from build123d import *

# Parameters (mm, degrees)
PAD015_DEPTH    = 1
PAD016_DEPTH    = 3
SKETCH029_R     = 1.6
POCKET012_DEPTH = 5


with BuildPart() as part:
    # Sketch027 → Pad015 (new body)
    with BuildSketch(Plane.XY):
        with BuildLine():
            Line((-54.625, 46.125), (-54.625, -46.125))
            ThreePointArc((-54.625, -46.125), (-54.332107, -46.832107), (-53.625, -47.125))
            Line((-53.625, -47.125), (53.625, -47.125))
            ThreePointArc((53.625, -47.125), (54.332107, -46.832107), (54.625, -46.125))
            Line((54.625, -46.125), (54.625, 46.125))
            ThreePointArc((54.625, 46.125), (54.332107, 46.832107), (53.625, 47.125))
            Line((53.625, 47.125), (-53.625, 47.125))
            ThreePointArc((-53.625, 47.125), (-54.332107, 46.832107), (-54.625, 46.125))
        make_face()
    extrude(amount=PAD015_DEPTH)

    # Sketch028 → Pad016 (join)
    with BuildSketch(Plane.XY):
        with BuildLine():
            Line((-54.625, 46.125), (-54.625, -46.125))
            ThreePointArc((-54.625, -46.125), (-54.332107, -46.832107), (-53.625, -47.125))
            Line((-53.625, -47.125), (53.625, -47.125))
            ThreePointArc((53.625, -47.125), (54.332107, -46.832107), (54.625, -46.125))
            Line((54.625, -46.125), (54.625, 46.125))
            ThreePointArc((54.625, 46.125), (54.332107, 46.832107), (53.625, 47.125))
            Line((53.625, 47.125), (-53.625, 47.125))
            ThreePointArc((-53.625, 47.125), (-54.332107, 46.832107), (-54.625, 46.125))
        make_face()
        with BuildLine():
            Line((-53.625, 45.125), (-53.625, -45.125))
            ThreePointArc((-53.625, -45.125), (-53.332107, -45.832107), (-52.625, -46.125))
            Line((-52.625, -46.125), (52.625, -46.125))
            ThreePointArc((52.625, -46.125), (53.332107, -45.832107), (53.625, -45.125))
            Line((53.625, -45.125), (53.625, 45.125))
            ThreePointArc((53.625, 45.125), (53.332107, 45.832107), (52.625, 46.125))
            Line((52.625, 46.125), (-52.625, 46.125))
            ThreePointArc((-52.625, 46.125), (-53.332107, 45.832107), (-53.625, 45.125))
        make_face(mode=Mode.SUBTRACT)
    extrude(amount=-PAD016_DEPTH)

    # Sketch029 → Pocket012 (cut)
    with BuildSketch(Plane.XY):
        with Locations((-48.5, 40)):
            Circle(SKETCH029_R)
        with Locations((-30, 40)):
            Circle(SKETCH029_R)
        with Locations((30, 40)):
            Circle(SKETCH029_R)
        with Locations((-30, -42)):
            Circle(SKETCH029_R)
        with Locations((-48.5, -42)):
            Circle(SKETCH029_R)
        with Locations((30, -42)):
            Circle(SKETCH029_R)
        with Locations((48.5, -42)):
            Circle(SKETCH029_R)
    extrude(amount=POCKET012_DEPTH, mode=Mode.SUBTRACT)


with BuildPart() as part_1:
    # Body007 placement: moved
    add(part.part.moved(Location((0, 0, 36.1))))


solid = part_1.part
Can you work these out from the model? Positions are in its coordinate system, mm. A direction names the side the tool comes from. Give positions to 0.01 mm unless a question says otherwise; leave off trailing zeros. Write each loop counter-clockwise with the first axis right and the second up, starting at its lowest first coordinate (ties: lowest second). Pieces come first, ordered by that corner, then holes. Notation, with made-up numbers: (-38, 3.5) -> (-24, 3.5) arc R14 ccw to (-24, 22.5) -> close; hole circle Ø1 at (80, -28). An arc over 180 degrees is marked (long way). Answer as a JSON object with one key per item and string values. Group by question number.
Item 1: Suppose I cut it at B-B (y = -42). Please give me the cut outline in (x, z) (3 decimals), plus the area to 3 significant figures.
Item 2: I'm going to push flat-ended pins straight in: P1, Ø2.5, axis at x = -30, y = 40, coming from the +Z side; P2, Ø3.5, axis at x = -30, y = -42, coming from the -Z side. Where does each tip first touch, or does it pass through?
Item 3: Suppose I cut it at D-D (x = 4.5). Please give me the cut outline in (y, z) (3 decimals).
Item 4: We'd pull the mould along Y, two halves only. Please class faces 3 (the face through (-1, 1, 37.1)), 4 (the face through (49.24, -43.42, 36.59)), 5 (the face through (-1, -47.125, 35)), 6 (the face through (1, 47.125, 35)): +Y half, -Y half, draft (parallel to the pull), parting line (faces both ways), or undercut.
Item 5: Suppose I cut it at C-C (y = 36.5). Please give me the cut outline in (x, z) (3 decimals).
Item 6: Please list where these lines run through material, in increasing order: line 1 (Y direction, x = 30, z = 36.75) (3 decimals); line 2 (X direction, y = 40, z = 36.7) (3 decimals); line 3 (Y direction, x = 48.5, z = 36.35) (3 decimals). Write a range as [from, to].
Item 7: For faces 1 (the face through (53.625, -1, 35)), 2 (the face through (-31.27, 39.03, 36.59)), which set-ups out of +Z, -Z, +X, -X, +Y, -Y let a thin tool reach every point of the face, with its end or its side?
Item 8: Suppose I cut it at A-A (x = -48.5). Please give me the cut outline in (y, z) (3 decimals).
Findings:
{
 "1": {"outline": "(-54.625, 33.1) -> (-53.625, 33.1) -> (-53.625, 36.1) -> (-50.1, 36.1) -> (-50.1, 37.1) -> (-54.625, 37.1) -> close; (-46.9, 36.1) -> (-31.6, 36.1) -> (-31.6, 37.1) -> (-46.9, 37.1) -> close; (-28.4, 36.1) -> (28.4, 36.1) -> (28.4, 37.1) -> (-28.4, 37.1) -> close; (31.6, 36.1) -> (46.9, 36.1) -> (46.9, 37.1) -> (31.6, 37.1) -> close; (50.1, 36.1) -> (53.625, 36.1) -> (53.625, 33.1) -> (54.625, 33.1) -> (54.625, 37.1) -> (50.1, 37.1) -> close", "area": "102 mm²"},
 "2": {"P1": "passes through", "P2": "stops at z = 36.1"},
 "3": {"outline": "(-47.125, 33.1) -> (-46.125, 33.1) -> (-46.125, 36.1) -> (46.125, 36.1) -> (46.125, 33.1) -> (47.125, 33.1) -> (47.125, 37.1) -> (-47.125, 37.1) -> close"},
 "4": {"face 3": "draft", "face 4": "undercut", "face 5": "-Y half", "face 6": "+Y half"},
 "5": {"outline": "(-54.625, 33.1) -> (-53.625, 33.1) -> (-53.625, 36.1) -> (53.625, 36.1) -> (53.625, 33.1) -> (54.625, 33.1) -> (54.625, 37.1) -> (-54.625, 37.1) -> close"},
 "6": {"line 1": "y = [-47.125, -43.6], [-40.4, 38.4], [41.6, 47.125]", "line 2": "x = [-54.625, -50.1], [-46.9, -31.6], [-28.4, 28.4], [31.6, 54.625]", "line 3": "y = [-47.125, -43.6], [-40.4, 47.125]"},
 "7": {"face 1": "-Z", "face 2": "+Z, -Z"},
 "8": {"outline": "(-47.125, 33.1) -> (-46.125, 33.1) -> (-46.125, 36.1) -> (-43.6, 36.1) -> (-43.6, 37.1) -> (-47.125, 37.1) -> close; (-40.4, 36.1) -> (38.4, 36.1) -> (38.4, 37.1) -> (-40.4, 37.1) -> close; (41.6, 36.1) -> (46.125, 36.1) -> (46.125, 33.1) -> (47.125, 33.1) -> (47.125, 37.1) -> (41.6, 37.1) -> close"}
}
